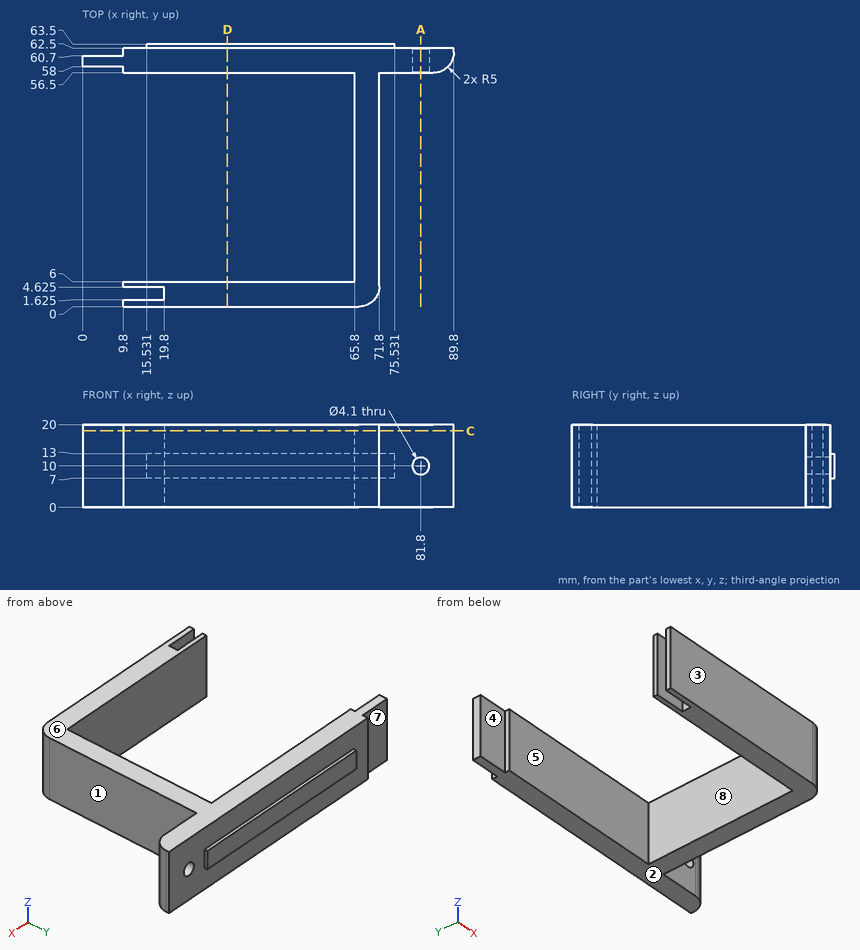
Drawing for the job (mm, zero at the part's lowest x, y, z). A direction names the side the tool comes from. Give positions to 0.01 mm unless a question says otherwise; leave off trailing zeros. Loops run counter-clockwise (first coordinate to the right, second up) from the corner with the lowest first, then second, coordinate; pieces in that order, holes last. Notation, with made-up numbers: M 18.25,32.25 L 51.25,32.25 A15 cw 51.25,40.25 Z; hole C 12.5,11.25 d11. An arc over 180 degrees is marked long. Use one line per item in the form item = value.
Item 1: Slice it at D-D (x = 35). List the corners of the cut face in (y, z), plus the area to 3 significant figures.
Determined:
outline = M 0,0 L 6,0 L 6,20 L 0,20 Z; M 56.5,0 L 62.5,0 L 62.5,7 L 63.5,7 L 63.5,13 L 62.5,13 L 62.5,20 L 56.5,20 Z
area = 246 mm2
Item 2: Drill centre lines: probe 1 along Y at (x, z) = (16.5, 15.25) (1 decimal); probe 2 along Y at (x, z) = (65.5, 11.5); probe 3 along Y at (x, z) = (39, 3.25). Where is each one in solid material? Low to high. Write a range as from..to.
Determined:
probe_1 = 0..1.6, 4.6..6, 56.5..62.5
probe_2 = 0..6, 56.5..63.5
probe_3 = 0..6, 56.5..62.5
Item 3: Which spindle directions (+Z, -Z, +X, -X, +Y, -Y) get a long thin tool onto all of the face, cutting with end or side? Do the marked faces 1, 2, 3, 4 and 5. Say none if no direction does.
Determined:
face_1 = +Z, -Z, +X, -Y
face_2 = -Z, +X, -X, +Y, -Y
face_3 = +Z, -Z, +X, -X, -Y
face_4 = +Z, -Z, -X, -Y
face_5 = +Z, -Z, -X
Item 4: Flat gauge pins, fed straight in: pin 1 (0.8 mm diameter, centred on y = 57.5, z = 10.5, fed in from -X); pin 2 (6.5 mm diameter, centred on x = 76.5, z = 12, fed in from -Y); pin 3 (5 mm diameter, centred on x = 12.5, z = 12, fed in from +Y). Where does each tip first touch, or does it go through?
Determined:
pin_1 = 9.8
pin_2 = 56.5
pin_3 = 62.5
Item 5: Slice it at C-C (z = 18.5). List the corners of the cut face in (x, y) (1 decimal), plus the area to 3 significant figures.
Determined:
outline = M 0,58 L 9.8,58 L 9.8,56.5 L 65.8,56.5 L 65.8,6 L 9.8,6 L 9.8,4.6 L 19.8,4.6 L 19.8,1.6 L 9.8,1.6 L 9.8,0 L 66.8,0 A5 ccw 71.8,5 L 71.8,56.5 L 84.8,56.5 A5 ccw 89.8,61.5 L 89.8,62.5 L 9.8,62.5 L 9.8,60.7 L 0,60.7 Z
area = 1,140 mm2
Item 6: Two-plate mould, pull along Y, no slides. Class the marked faces 6, 7 and 8: pulls with the +Y half, pulls with the -Y half, needs draft (parallel to the pull), parting line crosses it, or undercut.
Determined:
face_6 = needs draft
face_7 = pulls with the +Y half
face_8 = undercut
Item 7: Slice it at A-A (x = 81.8). List the corners of the cut face in (y, z).
Determined:
outline = M 56.5,0 L 62.5,0 L 62.5,7.95 L 56.5,7.95 Z; M 56.5,12.05 L 62.5,12.05 L 62.5,20 L 56.5,20 Z
